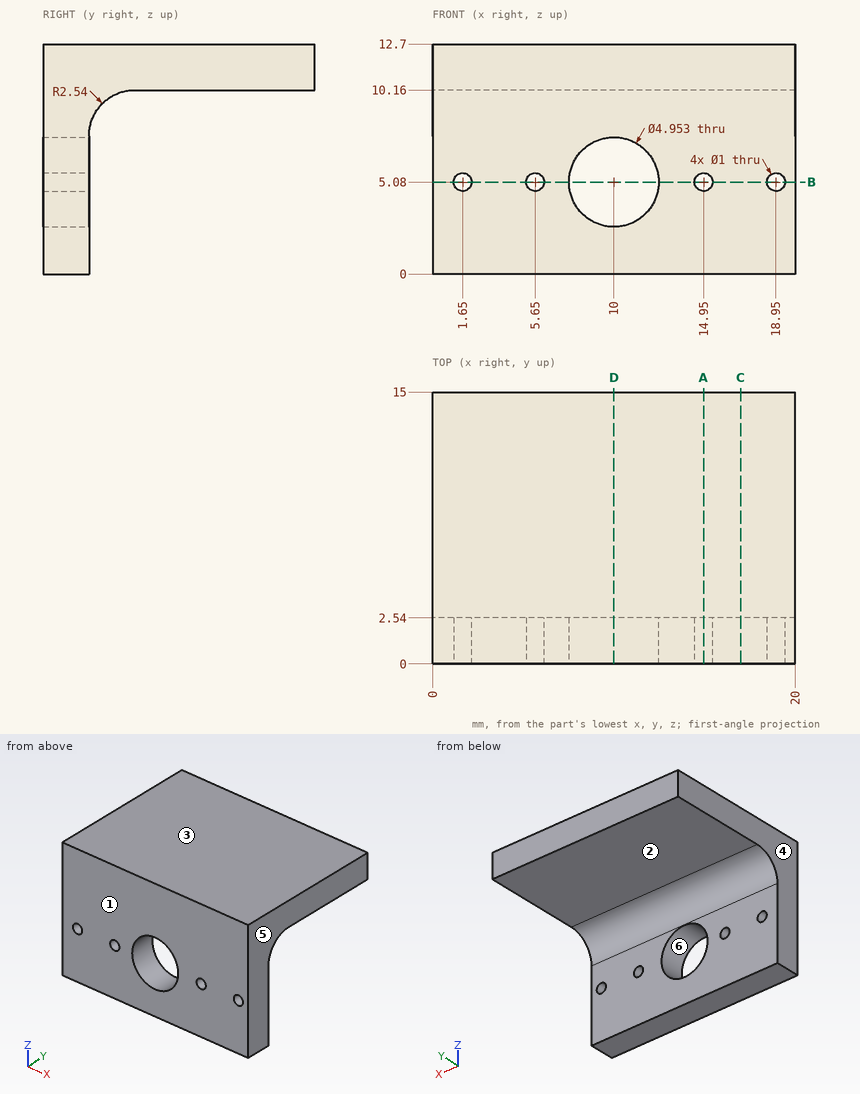
Geometry check sheet. Reference: drawing and pictorial views, mm from the part's lowest x, y, z. A direction names the side the tool comes from. Round coordinates to 2 decimals unless told otherwise and drop trailing zeros. Order: outer loops, then holes, each group sorted by start corner. A loop starts at its lowest first (then second) coordinate and runs counter-clockwise, first axis right, second up. Notation, with made-up numbers: M 52,-16.75 L 71,-16.75 A15 ccw 71,-3.75 Z; hole C 48,39 d1. An arc over 180 degrees is marked long. Answer in a Markdown table with one row per item.
(1) Scan lines: probe 1 along Z at (x, y) = (1.65, 1.45); probe 2 along Z at (x, y) = (10, 1.6); probe 3 along X at (y, z) = (2.5, 5.75). Record each from-to range of solid material in increasing order. Write a range as from..to.
Responses:
| item | result |
|---|---|
| probe 1 | z = 0..4.58, 5.58..12.7 |
| probe 2 | z = 0..2.6, 7.56..12.7 |
| probe 3 | x = 0..7.62, 12.38..20 |
(2) Tool access check on the marked faces 1 and 2. Record the directions out of +Z, -Z, +X, -X, +Y, -Y that give a thin tool (end or side, any length) a straight path to the whole face; none if there is none.
Responses:
| item | result |
|---|---|
| face 1 | +Z, -Z, +X, -X, -Y |
| face 2 | -Z, +X, -X, +Y |
(3) Go/stop test with a flat-tipped pin: P1, Ø5, axis at x = 5.5, y = 8.5, coming from the -Z side. Record where the tip stops, or that it passes through.
Responses:
| item | result |
|---|---|
| P1 | stops at z = 10.16 |
(4) Draft check along X on the marked faces 3, 4, 5 and 6. Enter one of: released by +X, released by -X, zero draft, split by the parting line, or undercut.
Responses:
| item | result |
|---|---|
| face 3 | zero draft |
| face 4 | released by -X |
| face 5 | released by +X |
| face 6 | undercut |
(5) Sectioned sample at B-B, the plane z = 5.08. Record the cut outline in (x, y), and give its area (3 significant figures).
Responses:
| item | result |
|---|---|
| outline | M 0,0 L 1.15,0 L 1.15,2.54 L 0,2.54 Z; M 2.15,0 L 5.15,0 L 5.15,2.54 L 2.15,2.54 Z; M 6.15,0 L 7.52,0 L 7.52,2.54 L 6.15,2.54 Z; M 12.48,0 L 14.45,0 L 14.45,2.54 L 12.48,2.54 Z; M 15.45,0 L 18.45,0 L 18.45,2.54 L 15.45,2.54 Z; M 19.45,0 L 20,0 L 20,2.54 L 19.45,2.54 Z |
| area | 28.1 mm² |
(6) Sectioned sample at A-A, the plane x = 14.95. Record the cut outline in (y, z), and give its area (3 significant figures).
Responses:
| item | result |
|---|---|
| outline | M 0,0 L 2.54,0 L 2.54,4.58 L 0,4.58 Z; M 0,5.58 L 2.54,5.58 L 2.54,7.62 A2.54 cw 5.08,10.16 L 15,10.16 L 15,12.7 L 0,12.7 Z |
| area | 62.8 mm² |
(7) Sectioned sample at D-D, the plane x = 10. Record the cut outline in (y, z), and give its area (3 significant figures).
Responses:
| item | result |
|---|---|
| outline | M 0,0 L 2.54,0 L 2.54,2.6 L 0,2.6 Z; M 0,7.56 L 2.54,7.56 L 2.54,7.62 A2.54 cw 5.08,10.16 L 15,10.16 L 15,12.7 L 0,12.7 Z |
| area | 52.7 mm² |
(8) Sectioned sample at C-C, the plane x = 17. Record the cut outline in (y, z).
Responses:
| item | result |
|---|---|
| outline | M 0,0 L 2.54,0 L 2.54,7.62 A2.54 cw 5.08,10.16 L 15,10.16 L 15,12.7 L 0,12.7 Z |
